Build history of the part. All positions in model axes, mm. Face numbers are marked on the shaded views. A direction names the side the tool comes from. Round coordinates to 2 decimals unless told otherwise and drop trailing zeros. Write each loop counter-clockwise with the first axis right and the second up, starting at its lowest first coordinate (ties: lowest second). Pieces come first, ordered by that corner, then holes.
1) Wall check: probe 1 along Y at (x, z) = (0, 1.9); probe 2 along X at (y, z) = (2.25, 0.8); probe 3 along Y at (x, z) = (-3.5, 5.7). Give the ranges that are in metal, low to high.
2) Saw through at A-A (y = 0). Write the cut outline in (x, z), plus the area to 3 significant figures.
3) Saw through at D-D (x = 4). Write the cut outline in (y, z), plus the area to 3 significant figures.
4) Which spindle directions (+Z, -Z, +X, -X, +Y, -Y) get a long thin tool onto all of the face, cutting with end or side? Do the marked faces 1, 2 and 3. Say none if no direction does.
5) Flat gauge pins, fed straight in: pin 1 (3 mm diameter, centred on y = 4, z = 5, fed in from +X); pin 2 (1.8 mm diameter, centred on x = 0, y = 0, fed in from +Z). Where does each tip first touch, or does it go through?
6) Pull direction X, two halves, no side cores. Call the marked faces 4, 5, 6 and 7: +X half, -X half, draft (parallel to the pull), parting line (faces both ways), or undercut.
7) Saw through at C-C (y = 2.75). Write the cut outline in (x, z), plus the area to 3 significant figures.
from build123d import *

# Parameters (mm, degrees)
F0_R     = 1.5
F1_DEPTH = 6


with BuildPart() as f1:
    # F0 (on Top) → F1 (new body)
    with BuildSketch(Plane.XY):
        with BuildLine():
            ThreePointArc((1.340637, 2.110141), (0.956709, 2.309699), (0.544121, 2.440068))
            ThreePointArc((0.544121, 2.440068), (0.599298, 3.627163), (0.453396, 4.80655))
            ThreePointArc((0.453396, 4.80655), (0.383688, 4.920608), (0.257701, 4.965279))
            Line((0.257701, 4.965279), (-0.257701, 4.965279))
            ThreePointArc((-0.257701, 4.965279), (-0.383688, 4.920608), (-0.453396, 4.80655))
            ThreePointArc((-0.453396, 4.80655), (-0.599298, 3.627163), (-0.544121, 2.440068))
            ThreePointArc((-0.544121, 2.440068), (-0.956709, 2.309699), (-1.340637, 2.110141))
            ThreePointArc((-1.340637, 2.110141), (-2.141024, 2.98856), (-3.078145, 3.719344))
            ThreePointArc((-3.078145, 3.719344), (-3.208087, 3.750704), (-3.32876, 3.693204))
            Line((-3.32876, 3.693204), (-3.693204, 3.32876))
            ThreePointArc((-3.693204, 3.32876), (-3.750704, 3.208087), (-3.719344, 3.078145))
            ThreePointArc((-3.719344, 3.078145), (-2.98856, 2.141024), (-2.110141, 1.340637))
            ThreePointArc((-2.110141, 1.340637), (-2.309699, 0.956709), (-2.440068, 0.544121))
            ThreePointArc((-2.440068, 0.544121), (-3.627163, 0.599298), (-4.80655, 0.453396))
            ThreePointArc((-4.80655, 0.453396), (-4.920608, 0.383688), (-4.965279, 0.257701))
            Line((-4.965279, 0.257701), (-4.965279, -0.257701))
            ThreePointArc((-4.965279, -0.257701), (-4.920608, -0.383688), (-4.80655, -0.453396))
            ThreePointArc((-4.80655, -0.453396), (-3.627163, -0.599298), (-2.440068, -0.544121))
            ThreePointArc((-2.440068, -0.544121), (-2.309699, -0.956709), (-2.110141, -1.340637))
            ThreePointArc((-2.110141, -1.340637), (-2.98856, -2.141024), (-3.719344, -3.078145))
            ThreePointArc((-3.719344, -3.078145), (-3.750704, -3.208087), (-3.693204, -3.32876))
            Line((-3.693204, -3.32876), (-3.32876, -3.693204))
            ThreePointArc((-3.32876, -3.693204), (-3.208087, -3.750704), (-3.078145, -3.719344))
            ThreePointArc((-3.078145, -3.719344), (-2.141024, -2.98856), (-1.340637, -2.110141))
            ThreePointArc((-1.340637, -2.110141), (-0.956709, -2.309699), (-0.544121, -2.440068))
            ThreePointArc((-0.544121, -2.440068), (-0.599298, -3.627163), (-0.453396, -4.80655))
            ThreePointArc((-0.453396, -4.80655), (-0.383688, -4.920608), (-0.257701, -4.965279))
            Line((-0.257701, -4.965279), (0.257701, -4.965279))
            ThreePointArc((0.257701, -4.965279), (0.383688, -4.920608), (0.453396, -4.80655))
            ThreePointArc((0.453396, -4.80655), (0.599298, -3.627163), (0.544121, -2.440068))
            ThreePointArc((0.544121, -2.440068), (0.956709, -2.309699), (1.340637, -2.110141))
            ThreePointArc((1.340637, -2.110141), (2.141024, -2.98856), (3.078145, -3.719344))
            ThreePointArc((3.078145, -3.719344), (3.208087, -3.750704), (3.32876, -3.693204))
            Line((3.32876, -3.693204), (3.693204, -3.32876))
            ThreePointArc((3.693204, -3.32876), (3.750704, -3.208087), (3.719344, -3.078145))
            ThreePointArc((3.719344, -3.078145), (2.98856, -2.141024), (2.110141, -1.340637))
            ThreePointArc((2.110141, -1.340637), (2.309699, -0.956709), (2.440068, -0.544121))
            ThreePointArc((2.440068, -0.544121), (3.627163, -0.599298), (4.80655, -0.453396))
            ThreePointArc((4.80655, -0.453396), (4.920608, -0.383688), (4.965279, -0.257701))
            Line((4.965279, -0.257701), (4.965279, 0.257701))
            ThreePointArc((4.965279, 0.257701), (4.920608, 0.383688), (4.80655, 0.453396))
            ThreePointArc((4.80655, 0.453396), (3.627163, 0.599298), (2.440068, 0.544121))
            ThreePointArc((2.440068, 0.544121), (2.309699, 0.956709), (2.110141, 1.340637))
            ThreePointArc((2.110141, 1.340637), (2.98856, 2.141024), (3.719344, 3.078145))
            ThreePointArc((3.719344, 3.078145), (3.750704, 3.208087), (3.693204, 3.32876))
            Line((3.693204, 3.32876), (3.32876, 3.693204))
            ThreePointArc((3.32876, 3.693204), (3.208087, 3.750704), (3.078145, 3.719344))
            ThreePointArc((3.078145, 3.719344), (2.141024, 2.98856), (1.340637, 2.110141))
        make_face()
        Circle(F0_R, mode=Mode.SUBTRACT)
    extrude(amount=F1_DEPTH)


solid = f1.part
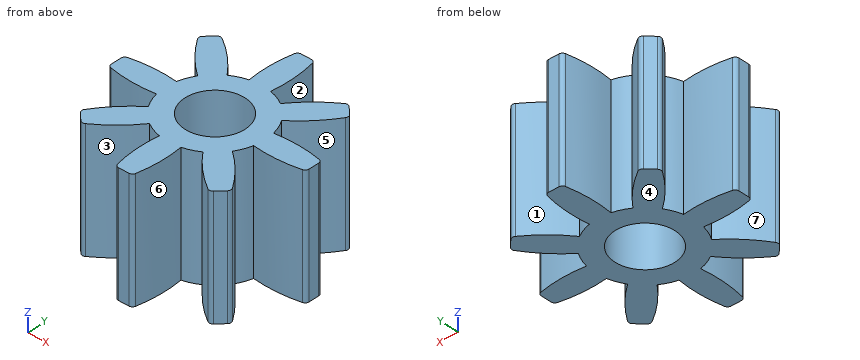
Evaluation:
1. probe 1: y = -4.97 to -1.5, 1.5 to 4.97
1. probe 2: x = -3.09 to -1.45, -1.09 to 1.09, 1.45 to 3.09
1. probe 3: y = -3.52 to -2.76, -0.6 to 0.6, 2.76 to 3.52
2. outline: (-4.97, 0) - (-1.5, 0) - (-1.5, 6) - (-4.97, 6) - close; (1.5, 0) - (4.97, 0) - (4.97, 6) - (1.5, 6) - close
2. area: 41.6 mm2
3. outline: (-0.58, 0) - (0.58, 0) - (0.58, 6) - (-0.58, 6) - close
3. area: 6.90 mm2
4. face 1: +Z, -Z, +Y
4. face 2: +Z, -Z
4. face 3: +Z, -Z, -Y
5. pin 1: stops at x = 3.75
5. pin 2: passes through
6. face 4: draft
6. face 5: +X half
6. face 6: undercut
6. face 7: -X half
7. outline: (-3.49, 0) - (-1.9, 0) - (-1.9, 6) - (-3.49, 6) - close; (-0.58, 0) - (0.58, 0) - (0.58, 6) - (-0.58, 6) - close; (1.9, 0) - (3.49, 0) - (3.49, 6) - (1.9, 6) - close
7. area: 26.1 mm2
